Autodesk Inventor part; units mm, degrees
ref_plane "YZ Plane" through (0, 0, 0) normal (1, 0, 0) x (0, 1, 0)
ref_plane "XZ Plane" through (0, 0, 0) normal (0, 1, 0) x (-1, 0, 0)
ref_plane "XY Plane" through (0, 0, 0) normal (0, 0, 1) x (1, 0, 0)
sketch "스케치1" plane through (0, 0, 0) normal (0, 0, 1) x (1, 0, 0)
  circle A0 centre (-7.7782, -7.7782) radius 1.55
  circle A1 centre (7.7782, -7.7782) radius 1.55
  circle A2 centre (7.7782, 7.7782) radius 1.55
  circle A3 centre (-7.7782, 7.7782) radius 1.55
  circle A4 centre (0, 0) radius 5
  circle A5 centre (0, 0) radius 13.9
  circle A6 centre (0, 11) radius 1.55
  circle A7 centre (11, 0) radius 1.55
  circle A8 centre (0, -11) radius 1.55
  circle A9 centre (-11, 0) radius 1.55
  line L0 (27.0238, -10.8065) -> (11.6088, -26.2214)
  line L1 (-10.8065, 27.0238) -> (-26.2214, 11.6088)
  line L2 (-10.8065, 27.0238) -> (-26.2214, 11.6088)
  line L3 (-10.8065, 27.0238) -> (-26.2214, 11.6088)
  line L4 (-26.2214, 11.6088) -> (11.6088, -26.2214)
  line L5 (11.6088, -26.2214) -> (27.0238, -10.8065)
  line L6 (27.0238, -10.8065) -> (-10.8065, 27.0238)
  line L7 (11.6795, -26.1507) -> (26.9531, -10.8772)
  line L8 (26.9531, -10.8772) -> (22.7104, -6.6345)
  line L9 (7.4369, -21.908) -> (22.7104, -6.6345)
  line L10 (11.6795, -26.1507) -> (7.4369, -21.908)
  circle A10 centre (0, 0) radius 7.5
  point P0 (0, 0)
  point P1 (-13.8807, -0.7318)
  point P2 (-0.7318, -13.8807)
  point P3 (13.6634, 2.554)
  point P4 (2.554, 13.6634)
extrude "돌출1" add sketch "스케치1" along normal blind 6 contours A0 L4 A5 L6 A2 | A0 L4 A5 | L4 L1 L6 A5 | A5 L6 L0 L8 L9 L10 L4 | A5 L6 A2 | L10 L9 L8 L0
sketch "스케치2" plane through (0, 0, 0) normal (0, 0, -1) x (-1, 0, 0)
  circle A0 centre (13.847, 19.7406) radius 1.35
  circle A1 centre (18.9382, 14.6494) radius 1.35
  circle A2 centre (-14.6494, -18.9382) radius 1.35
  circle A3 centre (-19.7406, -13.847) radius 1.35
  point P0 (0, 0)
extrude "돌출2" cut sketch "스케치2" against normal blind 6
properties part number "_arm_pti" material "PMMA 플라스틱"
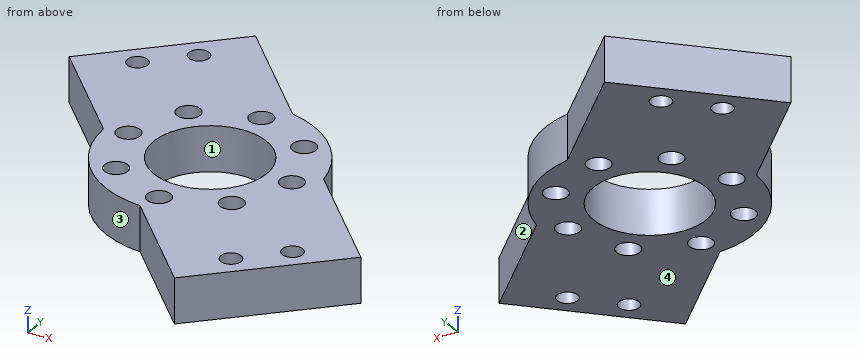
The listing builds one solid part. Answer for the finished solid, in the listing's coordinates (mm). Face numbers are marked on the shaded views. Coordinates: 2 decimals unless noted, no trailing zeros. Write each loop counter-clockwise with the first axis right and the second up, starting at its lowest first coordinate (ties: lowest second). Pieces come first, ordered by that corner, then holes. Notation, with made-up numbers: M 52,-12 L 78,-12 A12 cw 78,-2 Z; hole C 11,-22 d4. An arc over 180 degrees is marked long. Write each question's results on one line, items separated by ' | '.
Item 1: For a pull along Y with two mould halves and no side action, classify the marked faces 1, 2, 3 and 4 as released by +Y, released by -Y, zero draft, split by the parting line, or undercut.
Answer below:
face 1: undercut | face 2: released by +Y | face 3: released by -Y | face 4: zero draft
Item 2: Given P1, Ø2, axis at y = -11, z = 5, coming from the -X side, flat-ended and moving along its own axis, determine where the tip first touches the part or whether it passes through.
Answer below:
P1: x = -9.65
Item 3: The part is cut by section A-A on x = -19. Determine the outline of the cut face in (y, z).
Answer below:
outline: M 4.39,0 L 13.3,0 L 13.3,6 L 4.39,6 Z; M 16,0 L 18.83,0 L 18.83,6 L 16,6 Z
Item 4: The part is cut by section C-C on z = 4. State how many separate pieces and enclosed holes the cut face has, and give its area (3 significant figures).
Answer below:
separate pieces: 1 | enclosed holes: 13 | area: 978 mm2
Item 5: Consider probe 1 along X at (y, z) = (9, 5.3); probe 2 along X at (y, z) = (-9, 1.75); probe 3 along X at (y, z) = (-14, 1.8). Determine where each line is inside the solid, lowest interval first. Write a range as [from, to].
Answer below:
probe 1: [-23.61, -8.73], [-6.82, 6.82], [8.73, 10.59] | probe 2: [-10.59, -8.73], [-6.82, 6.82], [8.73, 25.22] | probe 3: [-0.61, 18.4], [21.08, 23.83]
Item 6: The part is cut by section D-D on x = 0.5. Determine the outline of the cut face in (y, z).
Answer below:
outline: M -15.11,0 L -12.47,0 L -12.47,6 L -15.11,6 Z; M -9.53,0 L -7.48,0 L -7.48,6 L -9.53,6 Z; M 7.48,0 L 9.53,0 L 9.53,6 L 7.48,6 Z; M 12.47,0 L 15.72,0 L 15.72,6 L 12.47,6 Z
Item 7: The part is cut by section B-B on y = 11. Determine the outline of the cut face in (x, z).
Answer below:
outline: M -25.61,0 L -1.55,0 L -1.55,6 L -25.61,6 Z; M 1.55,0 L 8.5,0 L 8.5,6 L 1.55,6 Z
